from build123d import *

# Parameters (mm, degrees)
SKETCH1_W           = 50.8
SKETCH1_H           = 76.2
SKETCH1_R           = 3.302
BOSS_EXTRUDE1_DEPTH = 25.4
SKETCH2_W           = 45.72
SKETCH2_H           = 20.32
CUT_EXTRUDE1_DEPTH  = 38.1
SKETCH3_R           = 1.5875
CUT_EXTRUDE2_DEPTH  = 26.4


with BuildPart() as part:
    # Sketch1 → Boss-Extrude1 (new body)
    with BuildSketch(Plane.XY):
        with Locations((25.4, 38.1)):
            Rectangle(SKETCH1_W, SKETCH1_H)
        with Locations((25.4, 13.208)):
            Circle(SKETCH1_R, mode=Mode.SUBTRACT)
        with Locations((25.4, 26.416)):
            Circle(SKETCH1_R, mode=Mode.SUBTRACT)
    extrude(amount=BOSS_EXTRUDE1_DEPTH)

    # Sketch2 → Cut-Extrude1 (cut)
    with BuildSketch(Plane(origin=(0, 76.2, 0), x_dir=(1, 0, 0), z_dir=(0, 1, 0))):
        with Locations((25.4, -12.7)):
            Rectangle(SKETCH2_W, SKETCH2_H)
    extrude(amount=-CUT_EXTRUDE1_DEPTH, mode=Mode.SUBTRACT)

    # Sketch3 → Cut-Extrude2 (cut, through all)
    with BuildSketch(Plane.XY.offset(25.4)):
        with Locations((25.4, 71.628)):
            Circle(SKETCH3_R)
    extrude(amount=-CUT_EXTRUDE2_DEPTH, mode=Mode.SUBTRACT)


solid = part.part
Input: part model. Units: mm. Frame: model coordinates. A direction names the side the tool comes from. Round coordinates to 2 decimals unless told otherwise and drop trailing zeros. Loops run counter-clockwise (first coordinate to the right, second up) from the corner with the lowest first, then second, coordinate; pieces in that order, holes last. Notation, with made-up numbers: (-0.75, 4.5) -> (38.25, 4.5) arc R17 ccw to (38.25, 9.5) -> close; hole circle Ø2 at (73.5, 51.25). An arc over 180 degrees is marked (long way). Answer as a JSON object with one key per item and string values. Group by question number.
1) Pin query (flat end, axial travel): pin 1 (19 mm diameter, centred on x = 21, y = 56.5, fed in from -Z); pin 2 (10 mm diameter, centred on x = 35, z = 13, fed in from +Y). Return the tip coordinate at first contact, or that it passes through.
2) Section query B-B on x = 15. Output: boundary loops of the cut face in (y, z).
3) Draft query along Z for faces 1 (the flat face through (25, 76.2, 2)), 2 (the flat face through (25, 39, 0)), 3 (the flat face through (2.54, 57, 13)). Return one class per face: +Z half, -Z half, draft (parallel to the pull), parting line (faces both ways), or undercut.
4) Section query C-C on y = 53.5. Output: boundary loops of the cut face in (x, z), plus the area to 3 significant figures.
5) Ray query, L1, parallel to X at y = 49, z = 19.25; L2, parallel to Z at x = 33, y = 62; L3, parallel to Y at x = 25.4, z = 11. Return the intervals inside material, ascending.
6) Section query A-A on x = 25.4. Output: boundary loops of the cut face in (y, z), plus the area to 3 significant figures.
7) Section query D-D on y = 28.5. Output: boundary loops of the cut face in (x, z), plus the area to 3 significant figures.
8) Reachability of faces 4 (the cylindrical face through (22.966, 15.44, 12.522)), 5 (the flat face through (48.26, 57, 13)) from +Z, -Z, +X, -X, +Y, -Y: full face, straight path, thin tool, end or side. Return the list, or none.
Reply:
{
 "1": {"pin 1": "stops at z = 0", "pin 2": "stops at y = 38.1"},
 "2": {"outline": "(0, 0) -> (76.2, 0) -> (76.2, 2.54) -> (38.1, 2.54) -> (38.1, 22.86) -> (76.2, 22.86) -> (76.2, 25.4) -> (0, 25.4) -> close"},
 "3": {"face 1": "draft", "face 2": "-Z half", "face 3": "undercut"},
 "4": {"outline": "(0, 0) -> (50.8, 0) -> (50.8, 25.4) -> (0, 25.4) -> close; hole (2.54, 2.54) -> (48.26, 2.54) -> (48.26, 22.86) -> (2.54, 22.86) -> close", "area": "361 mm2"},
 "5": {"L1": "x = 0 to 2.54, 48.26 to 50.8", "L2": "z = 0 to 2.54, 22.86 to 25.4", "L3": "y = 0 to 9.91, 16.51 to 23.11, 29.72 to 38.1"},
 "6": {"outline": "(0, 0) -> (9.91, 0) -> (9.91, 25.4) -> (0, 25.4) -> close; (16.51, 0) -> (23.11, 0) -> (23.11, 25.4) -> (16.51, 25.4) -> close; (29.72, 0) -> (70.04, 0) -> (70.04, 2.54) -> (38.1, 2.54) -> (38.1, 22.86) -> (70.04, 22.86) -> (70.04, 25.4) -> (29.72, 25.4) -> close; (73.22, 0) -> (76.2, 0) -> (76.2, 2.54) -> (73.22, 2.54) -> close; (73.22, 22.86) -> (76.2, 22.86) -> (76.2, 25.4) -> (73.22, 25.4) -> close", "area": "810 mm2"},
 "7": {"outline": "(0, 0) -> (22.84, 0) -> (22.84, 25.4) -> (0, 25.4) -> close; (27.96, 0) -> (50.8, 0) -> (50.8, 25.4) -> (27.96, 25.4) -> close", "area": "1,160 mm2"},
 "8": {"face 4": "+Z, -Z", "face 5": "+Y"}
}
